Geometry: final body of the model. Coordinates: model frame, mm. Face numbers are marked on the shaded views. A direction names the side the tool comes from. Give positions to 0.01 mm unless a question says otherwise; leave off trailing zeros. Write each loop counter-clockwise with the first axis right and the second up, starting at its lowest first coordinate (ties: lowest second). Pieces come first, ordered by that corner, then holes. Notation, with made-up numbers: (24.25, 4.25) - (56.25, 4.25) arc R31 ccw to (56.25, 41.25) - close; hole circle Ø11 at (-8.75, 6.25). An arc over 180 degrees is marked (long way). Return JSON: item names as keys, results as strings.
from build123d import *

# Parameters (mm, degrees)
CROQUIS1_W              = 5
CROQUIS1_H              = 3
SALIENTE_EXTRUIR1_DEPTH = 3


with BuildPart() as part:
    # Croquis1 → Saliente-Extruir1 (new body)
    with BuildSketch(Plane(origin=(0, 0, 0), x_dir=(1, 0, 0), z_dir=(0, 1, 0))):
        Polygon((4, 10), (4, 13), (0, 13), (0, 3), (2.5, 3), (2.5, 0), (12.5, 0), (12.5, 3), (18, 3), (18, 5), (15, 5), (15, 6.5), (15, 8), (18, 8), (18, 10), (14, 10), (9, 10), align=None)
        with Locations((11.5, 11.5)):
            Rectangle(CROQUIS1_W, CROQUIS1_H)
    extrude(amount=SALIENTE_EXTRUIR1_DEPTH)


solid = part.part
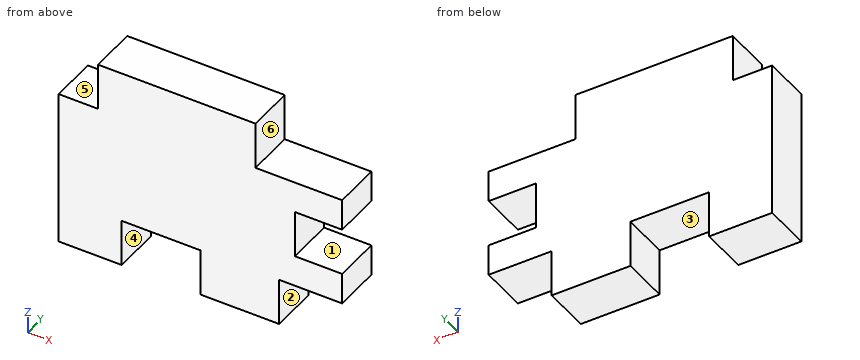
Q1. Section query D-D, the plane z = -1.25. Return the cut outline in (x, y), plus the area to 3 significant figures.
Answer key:
{"outline": "(2.5, 0) - (12.5, 0) - (12.5, 3) - (2.5, 3) - close", "area": "30.0 mm^2"}
Q2. Section query A-A, the plane x = 16.5. Return the cut outline in (y, z), plus the area to 3 significant figures.
Answer key:
{"outline": "(0, -10) - (3, -10) - (3, -8) - (0, -8) - close; (0, -5) - (3, -5) - (3, -3) - (0, -3) - close", "area": "12.0 mm^2"}
Q3. Set-up query: the marked faces 4, 5 and 6. Return all of +Z, -Z, +X, -X, +Y, -Y with unobstructed straight access to the full face (end or side cutting, diameter ignored); none if empty.
Answer key:
{"face 4": "-Z, +Y, -Y", "face 5": "+Z, -X, +Y, -Y", "face 6": "+Z, +X, +Y, -Y"}
Q4. Material intervals for probe 1 along X at (y, z) = (2.65, -12.25); probe 2 along Z at (x, y) = (7, 1.15); probe 3 along X at (y, z) = (0.7, -7), sorted ascending. Write a range as [from, to].
Answer key:
{"probe 1": "x = [0, 4], [9, 14]", "probe 2": "z = [-10, 0]", "probe 3": "x = [0, 15]"}
Q5. Pin query (flat end, axial travel): P1, Ø1, axis at y = 1.5, z = -1.5, coming from the +X side; P2, Ø1.5, axis at x = 14, y = 1, coming from the +Z side; P3, Ø0.9, axis at x = 16, y = 1.5, coming from the -Z side. Return the tip coordinate at first contact, or that it passes through.
Answer key:
{"P1": "stops at x = 12.5", "P2": "stops at z = -3", "P3": "stops at z = -10"}
Q6. Section query B-B, the plane z = -11. Return the cut outline in (x, y).
Answer key:
{"outline": "(0, 0) - (4, 0) - (4, 3) - (0, 3) - close; (9, 0) - (14, 0) - (14, 3) - (9, 3) - close"}
Q7. Mould query, pull axis X, two halves, no side actions, for the marked faces 1, 2 and 3. Classes: pulls with the +X half, pulls with the -X half, needs draft (parallel to the pull), parting line crosses it, or undercut.
Answer key:
{"face 1": "needs draft", "face 2": "pulls with the +X half", "face 3": "undercut"}
Q8. Section query C-C, the plane y = 0.5. Return the cut outline in (x, z), plus the area to 3 significant figures.
Answer key:
{"outline": "(0, -13) - (4, -13) - (4, -10) - (9, -10) - (9, -13) - (14, -13) - (14, -10) - (18, -10) - (18, -8) - (15, -8) - (15, -5) - (18, -5) - (18, -3) - (12.5, -3) - (12.5, 0) - (2.5, 0) - (2.5, -3) - (0, -3) - close", "area": "174 mm^2"}
